Verification items for this drawing (mm, ordinates from the low corner). A direction names the side the tool comes from. Round coordinates to 2 decimals unless told otherwise and drop trailing zeros. Order: outer loops, then holes, each group sorted by start corner. A loop starts at its lowest first (then second) coordinate and runs counter-clockwise, first axis right, second up. Notation, with made-up numbers: (17, -27.5) - (66, -27.5) arc R11 cw to (66, -18.5) - close; hole circle Ø5 at (72, 2.25). An arc over 180 degrees is marked (long way). Use a Markdown table: item, result. Add a question column.
(1) Mould release check, pull along Y, two halves, no side actions. Record for the marked faces 1, 2 and 3: released by +Y, released by -Y, zero draft, split by the parting line, or undercut.
(2) Section check A-A on x = 16. Record the boundary of the cut face in (y, z).
(3) Section check D-D on z = 4. Record the boundary of the cut face in (x, y).
(4) Thickness scan on line 1 along X through (y, z) = (24, 8.25) (1 decimal); line 2 along Y through (x, z) = (23.5, 9) (1 decimal); line 3 along Z through (x, y) = (20, 28). Record the ranges inside material, lowest first. Write a range as [from, to].
(5) Gauge pin test, flat ends, axial feed: P1, Ø4.5, axis at x = 24.84, y = 24.84, coming from the +Z side; P2, Ø7.5, axis at x = 7.16, y = 7.16, coming from the -Z side; P3, Ø4, axis at x = 14.5, z = 4, coming from the +Y side; P4, Ø3, axis at x = 16, z = 4, coming from the -Y side. Record the tip position at first contact, or that the pin passes through.
(6) Section check B-B on y = 15. Record the boundary of the cut face in (x, z).
(7) Section check C-C on y = 8.5. Record the boundary of the cut face in (x, z).
(8) Access from +Z, -Z, +X, -X, +Y, -Y to the whole of each face (thin tool, end or side, straight path). Record for the marked faces 4, 5, 6 and 7.
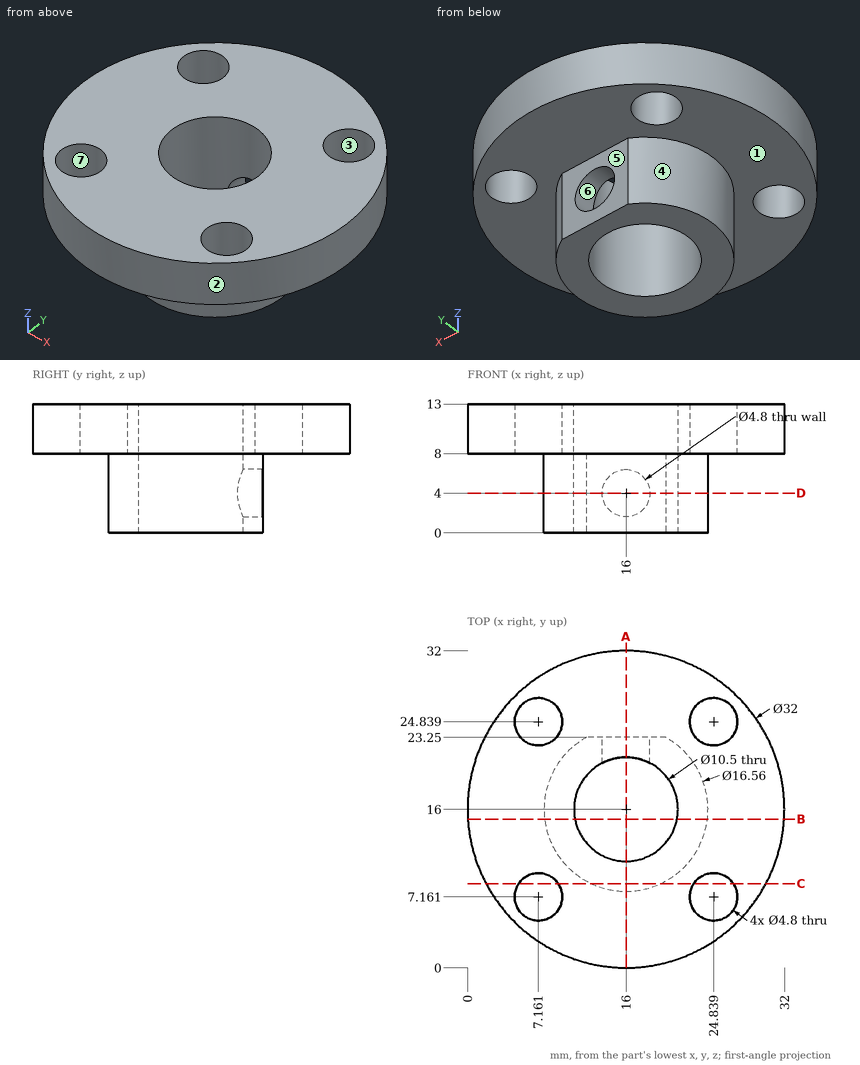
Check sheet entries:
| question | item | result |
|---|---|---|
| 1 | face 1 | zero draft |
| 1 | face 2 | split by the parting line |
| 1 | face 3 | undercut |
| 2 | outline | (0, 8) - (7.72, 8) - (7.72, 0) - (10.75, 0) - (10.75, 13) - (0, 13) - close; (21.25, 0) - (23.25, 0) - (23.25, 1.6) - (21.25, 1.6) - close; (21.25, 6.4) - (23.25, 6.4) - (23.25, 8) - (32, 8) - (32, 13) - (21.25, 13) - close |
| 3 | outline | (12, 23.25) arc R8.28 ccw (long way) to (20, 23.25) - (18.4, 23.25) - (18.4, 20.67) arc R5.25 cw (long way) to (13.6, 20.67) - (13.6, 23.25) - close |
| 4 | line 1 | x = [2.1, 4.9], [9.4, 22.6], [27.1, 29.9] |
| 4 | line 2 | y = [1.9, 5.2], [9.2, 22.8], [26.8, 30.1] |
| 4 | line 3 | z = [8, 13] |
| 5 | P1 | passes through |
| 5 | P2 | stops at z = 8 |
| 5 | P3 | stops at y = 23.25 |
| 5 | P4 | stops at y = 7.72 |
| 6 | outline | (0.03, 8) - (7.78, 8) - (7.78, 0) - (10.85, 0) - (10.85, 13) - (0.03, 13) - close; (21.15, 0) - (24.22, 0) - (24.22, 8) - (31.97, 8) - (31.97, 13) - (21.15, 13) - close |
| 7 | outline | (1.87, 8) - (5.17, 8) - (5.17, 13) - (1.87, 13) - close; (9.15, 8) - (12.49, 8) - (12.49, 0) - (19.51, 0) - (19.51, 8) - (22.85, 8) - (22.85, 13) - (9.15, 13) - close; (26.83, 8) - (30.13, 8) - (30.13, 13) - (26.83, 13) - close |
| 8 | face 4 | -Z |
| 8 | face 5 | -Z, +X, -X, +Y |
| 8 | face 6 | +Y |
| 8 | face 7 | +Z, -Z |
